```python
from build123d import *

# Parameters (mm, degrees)
F1_DEPTH       = 25.4
F2_R           = 76.2
F3_DEPTH       = 25.4
F5_D           = 17.4752
F5_CSINK_D     = 30.1752
F5_CSINK_ANGLE = 82


with BuildPart() as f1:
    # F0 (on Top) → F1 (new body)
    with BuildSketch(Plane.XY):
        with BuildLine():
            ThreePointArc((533.4, 0), (0, 533.4), (-533.4, 0))
            Line((-533.4, 0), (-381, 0))
            ThreePointArc((-381, 0), (0, 381), (381, 0))
            Line((381, 0), (533.4, 0))
        make_face()
    extrude(amount=F1_DEPTH)

    # F2 (on face) → F3 (join)
    with BuildSketch(Plane.XY.offset(25.4)):
        with Locations((-450.85, 75.9349557187)):
            Circle(F2_R)
        with Locations((450.85, 75.9349557187)):
            Circle(F2_R)
    extrude(amount=F3_DEPTH)

    # F5 (through all)
    with Locations(Plane(origin=(0, 0, 0), x_dir=(1, 0, 0), z_dir=(0, 0, -1))):
        with Locations((-407.0116534822, -206.7221845356), (-231.690010169, -393.0945802086), (16.3125792691, -456.0792141678), (259.3174608987, -375.9482214927), (421.2113483751, -177.8)):
            CounterSinkHole(F5_D / 2, F5_CSINK_D / 2, counter_sink_angle=F5_CSINK_ANGLE)


solid = f1.part
```
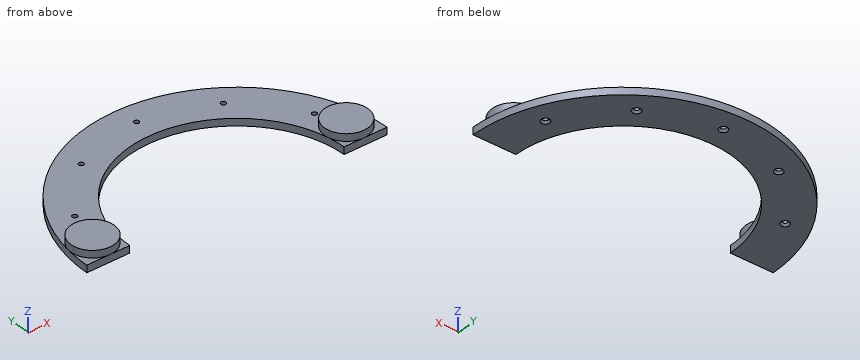
Input: part model. Units: mm. Frame: model coordinates. Round coordinates to 2 decimals unless told otherwise and drop trailing zeros. Loops run counter-clockwise (first coordinate to the right, second up) from the corner with the lowest first, then second, coordinate; pieces in that order, holes last. Notation, with made-up numbers: M 5,47 L 11,47 A18 ccw 11,77 Z; hole C 44.25,73 d2. An arc over 180 degrees is marked long. Answer in a Markdown table with one row per item. Add a question column.
1. Section B-B (y = 240.5). Output: boundary loops of the cut face in (x, z), and give its area (3 significant figures).
2. Section C-C (x = 82.5). Output: boundary loops of the cut face in (y, z), and give its area (3 significant figures).
3. Ray query, probe 1 along X at (y, z) = (177.8, 20); probe 2 along Z at (x, y) = (346.5, 181); probe 3 along X at (y, z) = (201.5, 7). Return the intervals inside material, ascending.
4. Section A-A (y = 101). Output: boundary loops of the cut face in (x, z), and give its area (3 significant figures).
5. Contact query for flat-ended pins moving along their axis: pin 1 (15.5 mm diameter, centred on x = 421.21, y = 177.8, fed in from +Z); pin 2 (2 mm diameter, centred on x = 375.5, y = 362, fed in from -Z); pin 3 (20 mm diameter, centred on x = -231.69, y = 393.09, fed in from +Z); pin 4 (8 mm diameter, centred on y = 365.5, z = 10.5, fed in from -X). Output: stop coordinate, or through.
6. Section D-D (x = 212). Output: boundary loops of the cut face in (y, z).
Values follow:
| question | item | result |
|---|---|---|
| 1 | outline | M -476.1,0 L -295.5,0 L -295.5,25.4 L -476.1,25.4 Z; M 295.5,0 L 476.1,0 L 476.1,25.4 L 295.5,25.4 Z |
| 1 | area | 9,170 mm^2 |
| 2 | outline | M 371.96,0 L 526.98,0 L 526.98,25.4 L 371.96,25.4 Z |
| 2 | area | 3,940 mm^2 |
| 3 | probe 1 | -502.89 to -336.97, 336.97 to 412.47, 429.95 to 502.89 |
| 3 | probe 2 | 0 to 25.4 |
| 3 | probe 3 | -493.88 to -414.34, -399.68 to -323.36, 323.36 to 493.88 |
| 4 | outline | M -523.75,0 L -367.37,0 L -367.37,25.4 L -378.89,25.4 L -378.89,50.8 L -522.81,50.8 L -522.81,25.4 L -523.75,25.4 Z; M 367.37,0 L 523.75,0 L 523.75,25.4 L 522.81,25.4 L 522.81,50.8 L 378.89,50.8 L 378.89,25.4 L 367.37,25.4 Z |
| 4 | area | 15,300 mm^2 |
| 5 | pin 1 | through |
| 5 | pin 2 | z = 0 |
| 5 | pin 3 | z = 25.4 |
| 5 | pin 4 | x = -392.22 |
| 6 | outline | M 316.57,0 L 489.46,0 L 489.46,25.4 L 316.57,25.4 Z |
